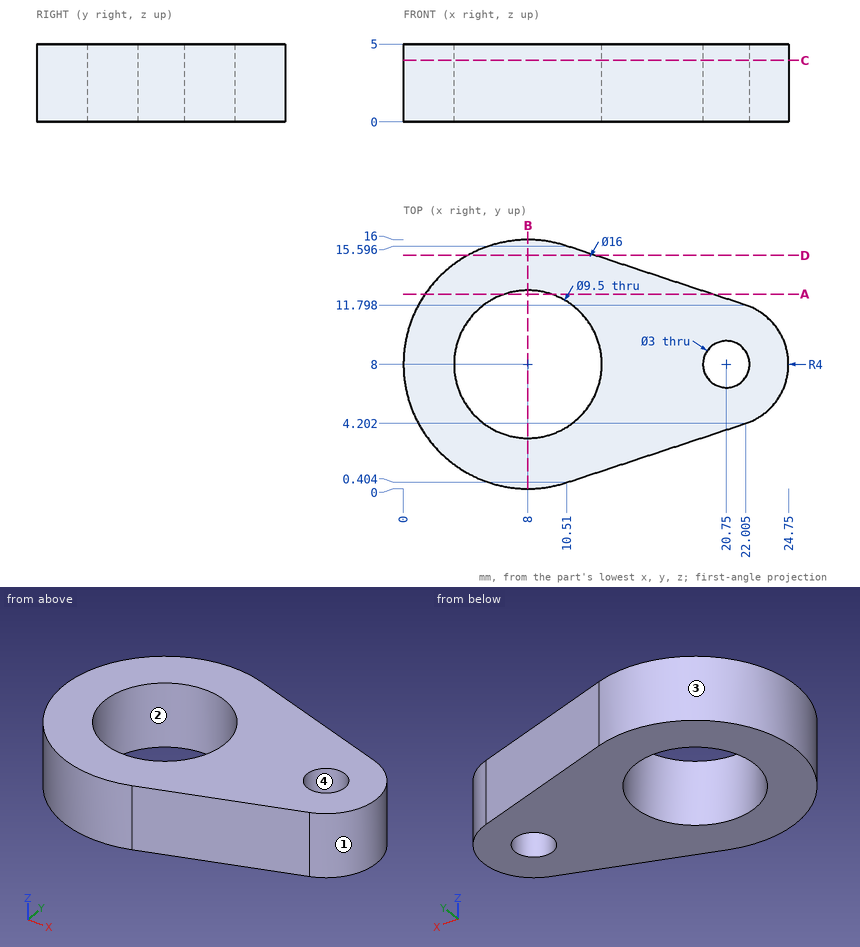
Geometry check sheet. Reference: drawing and pictorial views, mm from the part's lowest x, y, z. Give positions to 0.01 mm unless a question says otherwise; leave off trailing zeros. Order: outer loops, then holes, each group sorted by start corner. A loop starts at its lowest first (then second) coordinate and runs counter-clockwise, first axis right, second up.
1. Section check C-C, the plane z = 3.95. Give the number of separate pieces and of enclosed holes in the cut face, and give its area (3 significant figures).
2. Gauge pin test, flat end, axial feed: pin 1 Ø1 at (x, z) = (16, 2.5) entering from -Y. Record the tip position at first contact, or that the pin passes through.
3. Section check D-D, the plane y = 15. Enter the section's corners in (x, z), and give its area (3 significant figures).
4. Release check for a two-part mould opening along X. For the marked faces 1, 2, 3 and 4 record: pulls with the +X half, pulls with the -X half, needs draft (parallel to the pull), parting line crosses it, or undercut.
5. Section check A-A, the plane y = 12.5. Enter the section's corners in (x, z).
6. Thickness scan on L1, parallel to Y at x = 8, z = 1.25; L2, parallel to X at y = 7.75, z = 2.85; L3, parallel to Y at x = 20.5, z = 0.8 (1 decimal). Record the ranges inside material, lowest first.
7. Section check B-B, the plane x = 8. Enter the section's corners in (y, z), and give its area (3 significant figures).
Values follow:
1. separate pieces: 1
1. enclosed holes: 2
1. area: 208 mm2
2. pin 1: stops at y = 2.05
3. outline: (4.13, 0) - (12.31, 0) - (12.31, 5) - (4.13, 5) - close
3. area: 40.9 mm2
4. face 1: pulls with the +X half
4. face 2: undercut
4. face 3: parting line crosses it
4. face 4: undercut
5. outline: (1.39, 0) - (6.48, 0) - (6.48, 5) - (1.39, 5) - close; (9.52, 0) - (19.88, 0) - (19.88, 5) - (9.52, 5) - close
6. L1: y = 0 to 3.25, 12.75 to 16
6. L2: x = 0 to 3.26, 12.74 to 19.27, 22.23 to 24.74
6. L3: y = 3.7 to 6.5, 9.5 to 12.3
7. outline: (0, 0) - (3.25, 0) - (3.25, 5) - (0, 5) - close; (12.75, 0) - (16, 0) - (16, 5) - (12.75, 5) - close
7. area: 32.5 mm2
